```python
from build123d import *

# Parameters (mm, degrees)
BOSS_EXTRU_2_DEPTH      = 6
ESQUISSE3_R             = 1.2
ENL_V_MAT_EXTRU_1_DEPTH = 6
ESQUISSE4_R             = 1.2
ENL_V_MAT_EXTRU_2_DEPTH = 6


with BuildPart() as part:
    # Esquisse2 → Boss.-Extru.2 (new body)
    with BuildSketch(Plane.XY):
        with BuildLine():
            Line((-1.2, 0), (-9.6, 0))
            Line((-9.6, 0), (-9.6, -1.2))
            Line((-9.6, -1.2), (-2.4, -1.2))
            ThreePointArc((-2.4, -1.2), (-1.551471863, -1.551471863), (-1.2, -2.4))
            Line((-1.2, -2.4), (-1.2, -9.6))
            Line((-1.2, -9.6), (0, -9.6))
            Line((0, -9.6), (0, -1.2))
            ThreePointArc((0, -1.2), (-0.351471863, -0.351471863), (-1.2, 0))
        make_face()
    extrude(amount=BOSS_EXTRU_2_DEPTH)

    # Esquisse3 → Enlèv. mat.-Extru.1 (cut)
    with BuildSketch(Plane(origin=(0, 0, 0), x_dir=(1, 0, 0), z_dir=(0, 1, 0))):
        with Locations(Location((-4.8, -3, 0), (0, 0, 270))):
            Circle(ESQUISSE3_R)
    extrude(amount=-ENL_V_MAT_EXTRU_1_DEPTH, mode=Mode.SUBTRACT)

    # Esquisse4 → Enlèv. mat.-Extru.2 (cut)
    with BuildSketch(Plane(origin=(0, 0, 0), x_dir=(0, 0, -1), z_dir=(1, 0, 0))):
        with Locations((-3, -4.8)):
            Circle(ESQUISSE4_R)
    extrude(amount=-ENL_V_MAT_EXTRU_2_DEPTH, mode=Mode.SUBTRACT)


solid = part.part
```
The listing builds one solid part. Answer for the finished solid, in the listing's coordinates (mm). A direction names the side the tool comes from. Coordinates: 2 decimals unless noted, no trailing zeros. Loops run counter-clockwise (first coordinate to the right, second up) from the corner with the lowest first, then second, coordinate; pieces in that order, holes last. Notation, with made-up numbers: M 74.25,28.5 L 92.25,28.5 A14 cw 92.25,50.5 Z; hole C 78.25,75 d7. An arc over 180 degrees is marked long. Answer as a JSON object with one key per item and string values. Group by question number.
Item 1: Which of the six approach directions +Z, -Z, +X, -X, +Y, -Y give full straight-line access (tool end or side, diameter ignored) to faces 1 (the face through (-0.342, -0.361, 2.958)), 2 (the face through (-1.2, -6, 2))?
Item 2: Section D-D (z = 1.5) is taken. Write down the section's boundary in (x, y), and give its area (3 significant figures).
Item 3: Determine the mould class of faces 3 (the face through (-3, -1, 0)), 4 (the face through (-0.59, -4.75, 4.2)), 5 (the face through (-9.6, -1, 3)) for opening direction Z: +Z half, -Z half, draft (parallel to the pull), parting line (faces both ways), or undercut.
Item 4: Section B-B (y = -4.8) is taken. Write down the section's boundary in (x, z), and give its area (3 significant figures).
Item 5: Consider L1, parallel to Y at x = -3.75, z = 2.1; L2, parallel to Y at x = -0.65, z = 3. Determine where each line is inside the solid, lowest interval first.
Item 6: Section A-A (z = 3) is taken. Write down the section's boundary in (x, y), and give its area (3 significant figures).
Item 7: Each of these flat-tipped pins is pushed along its axis until it touches: P1, Ø2, axis at x = -4, z = 2.5, coming from the +Y side; P2, Ø2, axis at y = -4, z = 4, coming from the -X side; P3, Ø2, axis at x = -4.8, z = 3, coming from the +Y side; P4, Ø1, axis at x = -3, z = 5, coming from the -Y side. Where does it stop, or does it pass through?
Solved:
{
 "1": {"face 1": "+Z, -Z, +X, +Y", "face 2": "+Z, -Z, -X, -Y"},
 "2": {"outline": "M -9.6,-1.2 L -2.4,-1.2 A1.2 cw -1.2,-2.4 L -1.2,-9.6 L 0,-9.6 L 0,-1.2 A1.2 ccw -1.2,0 L -9.6,0 Z", "area": "21.6 mm2"},
 "3": {"face 3": "-Z half", "face 4": "undercut", "face 5": "draft"},
 "4": {"outline": "M -1.2,0 L 0,0 L 0,1.8 L -1.2,1.8 Z; M -1.2,4.2 L 0,4.2 L 0,6 L -1.2,6 Z", "area": "4.32 mm2"},
 "5": {"L1": "y = -1.2 to 0", "L2": "y = -9.6 to -6, -3.6 to -0.13"},
 "6": {"outline": "M -9.6,-1.2 L -6,-1.2 L -6,0 L -9.6,0 Z; M -3.6,-1.2 L -2.4,-1.2 A1.2 cw -1.2,-2.4 L -1.2,-3.6 L 0,-3.6 L 0,-1.2 A1.2 ccw -1.2,0 L -3.6,0 Z; M -1.2,-9.6 L 0,-9.6 L 0,-6 L -1.2,-6 Z", "area": "15.8 mm2"},
 "7": {"P1": "stops at y = 0", "P2": "stops at x = -1.2", "P3": "passes through", "P4": "stops at y = -1.2"}
}
